Here's the drawing with two shaded views (mm, measured from the low corner). I have some questions. Round coordinates to 2 decimals unless told otherwise and drop trailing zeros. Loops run counter-clockwise (first coordinate to the right, second up) from the corner with the lowest first, then second, coordinate; pieces in that order, holes last. Notation, with made-up numbers: M 64,-30 L 90,-30 A18 cw 90,-11 Z; hole C 40.25,-7.5 d7. An arc over 180 degrees is marked long. Answer as a JSON object with one key per item and string values.
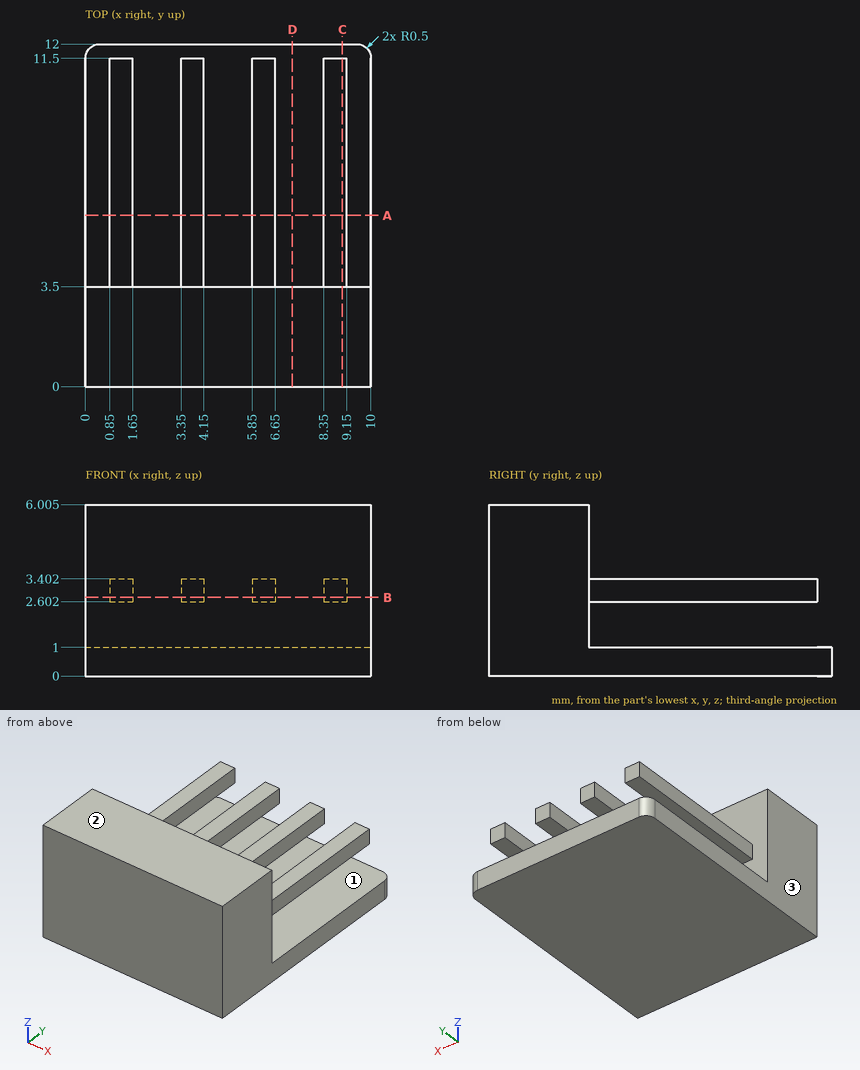
Item 1: I want a section at B-B on z = 2.75. List the corners of the cut face in (x, y) for me.
Solution:
{"outline": "M 0,0 L 10,0 L 10,3.5 L 9.15,3.5 L 9.15,11.5 L 8.35,11.5 L 8.35,3.5 L 6.65,3.5 L 6.65,11.5 L 5.85,11.5 L 5.85,3.5 L 4.15,3.5 L 4.15,11.5 L 3.35,11.5 L 3.35,3.5 L 1.65,3.5 L 1.65,11.5 L 0.85,11.5 L 0.85,3.5 L 0,3.5 Z"}
Item 2: If I drill on L1, parallel to X at y = 8.75, z = 3.25; L2, parallel to Y at x = 8, z = 4; L3, parallel to Z at x = 3.25, y = 8.25, over which ranges is the centre line in solid material (lowest first)? Write a range as from..to.
Solution:
{"L1": "x = 0.85..1.65, 3.35..4.15, 5.85..6.65, 8.35..9.15", "L2": "y = 0..3.5", "L3": "z = 0..1"}
Item 3: I want a section at C-C on x = 9. List the corners of the cut face in (y, z) for me (1 decimal).
Solution:
{"outline": "M 0,0 L 12,0 L 12,1 L 3.5,1 L 3.5,2.6 L 11.5,2.6 L 11.5,3.4 L 3.5,3.4 L 3.5,6 L 0,6 Z"}
Item 4: I want a section at A-A on y = 6. List the corners of the cut face in (x, z) for me.
Solution:
{"outline": "M 0,0 L 10,0 L 10,1 L 0,1 Z; M 0.85,2.6 L 1.65,2.6 L 1.65,3.4 L 0.85,3.4 Z; M 3.35,2.6 L 4.15,2.6 L 4.15,3.4 L 3.35,3.4 Z; M 5.85,2.6 L 6.65,2.6 L 6.65,3.4 L 5.85,3.4 Z; M 8.35,2.6 L 9.15,2.6 L 9.15,3.4 L 8.35,3.4 Z"}
Item 5: For P1, Ø0.6, axis at x = 1, y = 6, coming from the +Z side; P2, Ø0.9, axis at x = 1, z = 3, coming from the +Y side; P3, Ø1, axis at x = 5, z = 4, coming from the +Y side, each with a flat end and sliding along its axis, tell me the tip position at first contact or that it passes through.
Solution:
{"P1": "stops at z = 3.4", "P2": "stops at y = 11.5", "P3": "stops at y = 3.5"}
Item 6: I want a section at D-D on x = 7.25. List the corners of the cut face in (y, z) for me (1 decimal), plus the area to 3 significant figures.
Solution:
{"outline": "M 0,0 L 12,0 L 12,1 L 3.5,1 L 3.5,6 L 0,6 Z", "area": "29.5 mm2"}
Item 7: We'd pull the mould along Z, two halves only. Please class the marked faces 1, 2 and 3: +Z half, -Z half, draft (parallel to the pull), parting line (faces both ways), or undercut.
Solution:
{"face 1": "undercut", "face 2": "+Z half", "face 3": "draft"}
